CAD build for the part. Positions are in the model's coordinates, mm. A direction names the side the tool comes from. Give positions to 0.01 mm unless a question says otherwise; leave off trailing zeros. Loops run counter-clockwise (first coordinate to the right, second up) from the corner with the lowest first, then second, coordinate; pieces in that order, holes last. Notation, with made-up numbers: M 20.5,-21 L 30.5,-21 A22 cw 30.5,1 Z; hole C 74,75.5 d2. An arc over 180 degrees is marked long. Answer as CSV lines item,"result".
```python
from build123d import *

# Parameters (mm, degrees)
SKETCH_1_W                  = 120
SKETCH_1_H                  = 556
EXTRUDE_1_DEPTH             = 72
SHEET_START                 = 58.585786438
SHEET_METAL_1_DEPTH         = 2.914213562
SHEET_START_2               = -60
SHEET_METAL_1_2_DEPTH       = 118
SHEET_START_3               = 57.625
SHEET_METAL_1_3_DEPTH       = 0.960786438
SHEET_METAL_1_4_DEPTH       = 117.625
SHEET_METAL_1_5_OUTLINE_W   = 69.625
SHEET_METAL_1_5_OUTLINE_H   = 1.5
SHEET_METAL_1_5_OUTLINE_W_2 = 1.5
SHEET_METAL_1_5_OUTLINE_H_2 = 551.25
SHEET_METAL_1_5_DEPTH       = 0.375
SHEET_METAL_1_6_OUTLINE_W   = 69.625
SHEET_METAL_1_6_OUTLINE_H   = 1.5
SHEET_METAL_1_6_DEPTH       = 0.960786438
SHEET_START_4               = -276.585786438
SHEET_METAL_1_7_DEPTH       = 553.171572876
SHEET_START_5               = -275.625
SHEET_METAL_1_8_DEPTH       = 551.25
SHEET_METAL_1_9_OUTLINE_W   = 1.5
SHEET_METAL_1_9_OUTLINE_H   = 69.625
SHEET_METAL_1_9_DEPTH       = 553.171572876
SKETCH_6_R                  = 2
CUT_EXTRUDE_1_DEPTH         = 296.473772102


with BuildPart() as part:
    # Sketch 1 → 凸台-拉伸1 (new body)
    with BuildSketch(Plane(origin=(0, 0, 0), x_dir=(1, 0, 0), z_dir=(0, 1, 0))):
        Rectangle(SKETCH_1_W, SKETCH_1_H)
    extrude(amount=EXTRUDE_1_DEPTH)

    # Sheet Metal 1: read off the stored shape, not the designer's step
    # Sheet Metal 1 outline → Sheet Metal 1 (cut)
    with BuildSketch(Plane.YZ.offset(SHEET_START)):
        with BuildLine():
            Line((0, 279.5), (0, 276.585786438))
            Line((0, 276.585786438), (69.625, 276.585786438))
            Line((69.625, 276.585786438), (69.625, 275.625))
            Line((69.625, 275.625), (73.5, 275.625))
            Line((73.5, 275.625), (73.5, 276))
            ThreePointArc((73.5, 276), (72.474873734, 278.474873734), (70, 279.5))
            Line((70, 279.5), (69.625, 279.5))
            Line((69.625, 279.5), (0, 279.5))
        make_face()
        with BuildLine():
            Line((69.625, -276.585786438), (0, -276.585786438))
            Line((0, -276.585786438), (0, -279.5))
            Line((0, -279.5), (69.625, -279.5))
            Line((69.625, -279.5), (70, -279.5))
            ThreePointArc((70, -279.5), (72.474873734, -278.474873734), (73.5, -276))
            Line((73.5, -276), (73.5, -275.625))
            Line((73.5, -275.625), (69.625, -275.625))
            Line((69.625, -275.625), (69.625, -276.585786438))
        make_face()
    extrude(amount=SHEET_METAL_1_DEPTH, mode=Mode.SUBTRACT)

    # Sheet Metal 1 2 outline → Sheet Metal 1 2 (cut)
    with BuildSketch(Plane.YZ.offset(SHEET_START_2)):
        with BuildLine():
            Line((0, 278), (0, -278))
            Line((0, -278), (70, -278))
            ThreePointArc((70, -278), (71.414213562, -277.414213562), (72, -276))
            Line((72, -276), (72, 276))
            ThreePointArc((72, 276), (71.414213562, 277.414213562), (70, 278))
            Line((70, 278), (0, 278))
        make_face()
    extrude(amount=SHEET_METAL_1_2_DEPTH, mode=Mode.SUBTRACT)

    # Sheet Metal 1 3 outline → Sheet Metal 1 3 (cut)
    with BuildSketch(Plane.YZ.offset(SHEET_START_3)):
        Polygon((0, 278), (0, 276.585786438), (69.625, 276.585786438), (69.625, 275.625), (72, 275.625), (72, 278), align=None)
        Polygon((69.625, -276.585786438), (0, -276.585786438), (0, -278), (72, -278), (72, -275.625), (69.625, -275.625), align=None)
    extrude(amount=SHEET_METAL_1_3_DEPTH, mode=Mode.SUBTRACT)

    # Sheet Metal 1 4 outline → Sheet Metal 1 4 (add)
    with BuildSketch(Plane.YZ.offset(SHEET_START_2)):
        with BuildLine():
            Line((0, 279.5), (0, 278))
            Line((0, 278), (72, 278))
            Line((72, 278), (72, -278))
            Line((72, -278), (0, -278))
            Line((0, -278), (0, -279.5))
            Line((0, -279.5), (70, -279.5))
            ThreePointArc((70, -279.5), (72.474873734, -278.474873734), (73.5, -276))
            Line((73.5, -276), (73.5, 276))
            ThreePointArc((73.5, 276), (72.474873734, 278.474873734), (70, 279.5))
            Line((70, 279.5), (0, 279.5))
        make_face()
    extrude(amount=SHEET_METAL_1_4_DEPTH)

    # Sheet Metal 1 5 outline → Sheet Metal 1 5 (add)
    with BuildSketch(Plane.YZ.offset(SHEET_START_3)):
        with Locations((34.8125, 278.75)):
            Rectangle(SHEET_METAL_1_5_OUTLINE_W, SHEET_METAL_1_5_OUTLINE_H)
        with Locations((34.8125, -278.75)):
            Rectangle(SHEET_METAL_1_5_OUTLINE_W, SHEET_METAL_1_5_OUTLINE_H)
        with Locations((72.75, 0)):
            Rectangle(SHEET_METAL_1_5_OUTLINE_W_2, SHEET_METAL_1_5_OUTLINE_H_2)
    extrude(amount=SHEET_METAL_1_5_DEPTH)

    # Sheet Metal 1 6 outline → Sheet Metal 1 6 (add)
    with BuildSketch(Plane.YZ.offset(SHEET_START_3)):
        with Locations((34.8125, 278.75)):
            Rectangle(SHEET_METAL_1_6_OUTLINE_W, SHEET_METAL_1_6_OUTLINE_H)
        with Locations((34.8125, -278.75)):
            Rectangle(SHEET_METAL_1_6_OUTLINE_W, SHEET_METAL_1_6_OUTLINE_H)
    extrude(amount=SHEET_METAL_1_6_DEPTH)

    # Sheet Metal 1 7 outline → Sheet Metal 1 7 (cut)
    with BuildSketch(Plane.XY.offset(SHEET_START_4)):
        with BuildLine():
            Line((58, 0), (60, 0))
            Line((60, 0), (60, 70))
            ThreePointArc((60, 70), (59.414213562, 71.414213562), (58, 72))
            Line((58, 72), (58, 0))
        make_face()
    extrude(amount=SHEET_METAL_1_7_DEPTH, mode=Mode.SUBTRACT)

    # Sheet Metal 1 8 outline → Sheet Metal 1 8 (add)
    with BuildSketch(Plane.XY.offset(SHEET_START_5)):
        with BuildLine():
            Line((60, 0), (61.5, 0))
            Line((61.5, 0), (61.5, 70))
            ThreePointArc((61.5, 70), (60.474873734, 72.474873734), (58, 73.5))
            Line((58, 73.5), (58, 72))
            Line((58, 72), (60, 72))
            Line((60, 72), (60, 0))
        make_face()
    extrude(amount=SHEET_METAL_1_8_DEPTH)

    # Sheet Metal 1 9 outline → Sheet Metal 1 9 (add)
    with BuildSketch(Plane.XY.offset(SHEET_START_4)):
        with Locations((60.75, 34.8125)):
            Rectangle(SHEET_METAL_1_9_OUTLINE_W, SHEET_METAL_1_9_OUTLINE_H)
    extrude(amount=SHEET_METAL_1_9_DEPTH)

    # 草图6 → 切除-拉伸1 (cut, through all)
    with BuildSketch(Plane(origin=(0, 0, 0), x_dir=(1, 0, 0), z_dir=(0, 1, 0))):
        with Locations(Location((-43.5, -236.5, 0), (0, 0, 270))):
            Circle(SKETCH_6_R)
        with Locations(Location((31.5, -241.5, 0), (0, 0, 270))):
            Circle(SKETCH_6_R)
        with Locations(Location((-43.5, -116.5, 0), (0, 0, 270))):
            Circle(SKETCH_6_R)
        with Locations(Location((31.5, -71.5, 0), (0, 0, 270))):
            Circle(SKETCH_6_R)
        with Locations(Location((31.5, 71.5, 0), (0, 0, 90))):
            Circle(SKETCH_6_R)
        with Locations(Location((-43.5, 116.5, 0), (0, 0, 90))):
            Circle(SKETCH_6_R)
        with Locations(Location((31.5, 241.5, 0), (0, 0, 90))):
            Circle(SKETCH_6_R)
        with Locations(Location((-43.5, 236.5, 0), (0, 0, 90))):
            Circle(SKETCH_6_R)
    extrude(amount=CUT_EXTRUDE_1_DEPTH, mode=Mode.SUBTRACT)


solid = part.part
```
Q1. Cut at A-A (y = 60.5). Write the cut outline in (x, z).
Solution:
outline,"M -60,-279.5 L 58.59,-279.5 L 58.59,-278 L -60,-278 Z; M -60,278 L 58.59,278 L 58.59,279.5 L -60,279.5 Z; M 60,-276.59 L 61.5,-276.59 L 61.5,276.59 L 60,276.59 Z"
Q2. Pin check, flat tips, straight feed: P1, Ø3.5, axis at x = -43.5, z = 116.5, coming from the +Y side; P2, Ø0.5, axis at x = 60.5, z = -276.5, coming from the +Y side (3 decimals); P3, Ø6, axis at x = -1.5, z = 98.5, coming from the -Y side; P4, Ø6.5, axis at x = 31.5, z = -71.5, coming from the +Y side. Stop position of each tip, or through.
Solution:
P1,"passes through"
P2,"stops at y = 69.625"
P3,"stops at y = 72"
P4,"stops at y = 73.5"
Q3. Wall check: line 1 (Z direction, x = -24.5, y = 63.5); line 2 (Y direction, x = -35, z = 148); line 3 (X direction, y = 72.75, z = 116.5). Give the ranges that are in metal, low to high. Write a range as [from, to].
Solution:
line 1,"z = [-279.5, -278], [278, 279.5]"
line 2,"y = [72, 73.5]"
line 3,"x = [-60, -45.5], [-41.5, 60.17]"
Q4. Cut at B-B (x = -28). Write the cut outline in (y, z).
Solution:
outline,"M 0,-279.5 L 70,-279.5 A3.5 ccw 73.5,-276 L 73.5,276 A3.5 ccw 70,279.5 L 0,279.5 L 0,278 L 70,278 A2 cw 72,276 L 72,-276 A2 cw 70,-278 L 0,-278 Z"
Q5. Cut at C-C (z = 205). Write the cut outline in (x, y).
Solution:
outline,"M -60,72 L 58,72 A2 cw 60,70 L 60,0 L 61.5,0 L 61.5,70 A3.5 ccw 58,73.5 L -60,73.5 Z"
Q6. Which spindle directions (+Z, -Z, +X, -X, +Y, -Y) get a long thin tool onto all of the face, cutting with end or side? Do faces 1 (the flat face through (-2, 35, 278)), 2 (the flat face through (-2, 72, 4)), 3 (the flat face through (60, 35, -4)). Say none if no direction does.
Solution:
face 1,"+X, -X, -Y"
face 2,"-X, -Y"
face 3,"+Z, -Z, -X, -Y"
Q7. Mould opens along Z. For faces 4 (the flat face through (-2, 35, -279.5)), 5 (the flat face through (-2, 73.5, -4)), 6 (the flat face through (-2, 35, -278)) say: released by +Z, released by -Z, zero draft, split by the parting line, or undercut.
Solution:
face 4,"released by -Z"
face 5,"zero draft"
face 6,"undercut"
